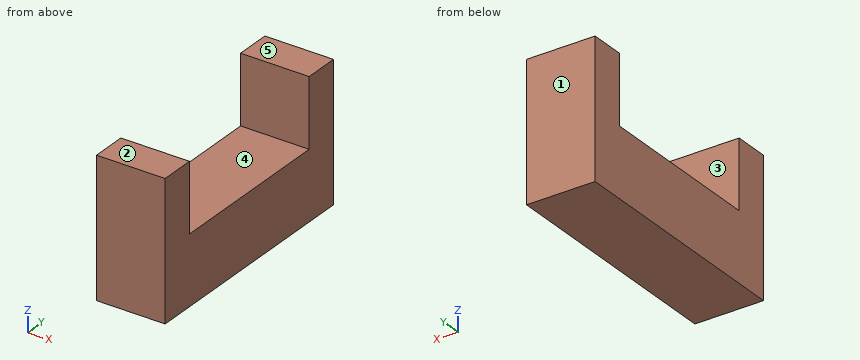
from build123d import *

# Parameters (mm, degrees)
F0_W     = 29.21
F0_H     = 57.15
F0_W_2   = 143.764
F1_DEPTH = 57.15


with BuildPart() as f1:
    # F0 (on Right) → F1 (new body)
    with BuildSketch(Plane.YZ):
        with Locations((158.369, 39.481787)):
            Rectangle(F0_W, F0_H)
        with Locations((158.369, -17.668213)):
            Rectangle(F0_W, F0_H)
        with Locations((71.882, -17.668213)):
            Rectangle(F0_W_2, F0_H)
        with Locations((-14.605, -17.668213)):
            Rectangle(F0_W, F0_H)
        with Locations((-14.605, 39.481787)):
            Rectangle(F0_W, F0_H)
    extrude(amount=F1_DEPTH)


solid = f1.part
Work out the finished part from the listing and answer in its coordinate system (mm). Face numbers are marked on the shaded views. A direction names the side the tool comes from. Give positions to 0.01 mm unless a question says otherwise; leave off trailing zeros. Loops run counter-clockwise (first coordinate to the right, second up) from the corner with the lowest first, then second, coordinate; pieces in that order, holes last. Notation, with made-up numbers: (83.5, 88.25) -> (102.5, 88.25) arc R15 cw to (102.5, 102.25) -> close; hole circle Ø5 at (-5, 82.25). An arc over 180 degrees is marked (long way). Use a Markdown table: item, result. Add a question column.
1) The part is cut by section A-A, the plane z = 42.5. Determine the outline of the cut face in (x, y), plus the area to 3 significant figures.
2) For a pull along Y with two mould halves and no side action, classify the marked faces 1, 2 and 3 as +Y half, -Y half, draft (parallel to the pull), parting line (faces both ways), or undercut.
3) Which of the six approach directions +Z, -Z, +X, -X, +Y, -Y give full straight-line access (tool end or side, diameter ignored) to the marked faces 4 and 5?
4) Each of these flat-tipped pins is pushed along its axis until it touches: P1, Ø8, axis at x = 48, y = 58, coming from the +Z side; P2, Ø3, axis at y = 66, z = -25.5, coming from the -X side. Where does it stop, or does it pass through?
5) Consider line 1 along Y through (x, z) = (35, 52.5); line 2 along Z through (x, y) = (30, 114). Determine where each line is inside the solid, lowest interval first.
6) The part is cut by section C-C, the plane y = 81. Determine the outline of the cut face in (x, z).
7) The part is cut by section B-B, the plane x = 10. Determine the outline of the cut face in (y, z), plus the area to 3 significant figures.
Reported:
| question | item | result |
|---|---|---|
| 1 | outline | (0, -29.21) -> (57.15, -29.21) -> (57.15, 0) -> (0, 0) -> close; (0, 143.76) -> (57.15, 143.76) -> (57.15, 172.97) -> (0, 172.97) -> close |
| 1 | area | 3,340 mm^2 |
| 2 | face 1 | +Y half |
| 2 | face 2 | draft |
| 2 | face 3 | undercut |
| 3 | face 4 | +Z, +X, -X |
| 3 | face 5 | +Z, +X, -X, +Y, -Y |
| 4 | P1 | stops at z = 10.91 |
| 4 | P2 | stops at x = 0 |
| 5 | line 1 | y = -29.21 to 0, 143.76 to 172.97 |
| 5 | line 2 | z = -46.24 to 10.91 |
| 6 | outline | (0, -46.24) -> (57.15, -46.24) -> (57.15, 10.91) -> (0, 10.91) -> close |
| 7 | outline | (-29.21, -46.24) -> (172.97, -46.24) -> (172.97, 68.06) -> (143.76, 68.06) -> (143.76, 10.91) -> (0, 10.91) -> (0, 68.06) -> (-29.21, 68.06) -> close |
| 7 | area | 14,900 mm^2 |
